Could you check a few things on this model? Use its own coordinates, in mm. A direction names the side the tool comes from. Give positions to 0.01 mm unless a question says otherwise; leave off trailing zeros. Order: outer loops, then holes, each group sorted by start corner. A loop starts at its lowest first (then second) coordinate and runs counter-clockwise, first axis right, second up. Notation, with made-up numbers: (24, 64) - (62, 64) arc R35 ccw to (62, 96) - close; hole circle Ø5 at (89.5, -22.75). An arc over 180 degrees is marked (long way). Put each result on its own line as item: value.
from build123d import *

# Parameters (mm, degrees)
SKETCH1_W           = 100
SKETCH1_H           = 40
BOSS_EXTRUDE1_DEPTH = 38
CUT_EXTRUDE2_START  = -12
SKETCH2_W           = 39.5
SKETCH2_H           = 34
CUT_EXTRUDE2_DEPTH  = 21
CUT_EXTRUDE4_REACH  = 81.36
SKETCH4_R           = 1.45
SKETCH6_W           = 100
SKETCH6_H           = 19
CUT_EXTRUDE5_DEPTH  = 87.215210375
FILLET1_R           = 0.5
CUT_EXTRUDE6_START  = 6.5
CUT_EXTRUDE6_DEPTH  = 0.5
CUT_EXTRUDE6_TAPER  = 2
CUT_EXTRUDE7_START  = 6.5
CUT_EXTRUDE7_DEPTH  = 0.5
CUT_EXTRUDE7_TAPER  = 2
CUT_EXTRUDE12_DEPTH = 9
CUT_EXTRUDE13_REACH = 72.385
SKETCH18_R          = 2.506862912
SKETCH18_R_2        = 2.693115416
SKETCH19_R          = 6.477
SKETCH19_R_2        = 4.572
CUT_EXTRUDE14_DEPTH = 0.79375


with BuildPart() as part:
    # Sketch1 → Boss-Extrude1 (new body)
    with BuildSketch(Plane.XY):
        with Locations((16.25, 1.5625)):
            Rectangle(SKETCH1_W, SKETCH1_H)
    extrude(amount=BOSS_EXTRUDE1_DEPTH)

    # Sketch2 → Cut-Extrude2 (cut)
    with BuildSketch(Plane(origin=(0, 0, 0), x_dir=(-1, 0, 0), z_dir=(0, 0, -1)).offset(CUT_EXTRUDE2_START)):
        with Locations((-38.5, 1.5625)):
            Rectangle(SKETCH2_W, SKETCH2_H)
        with Locations((6, 1.5625)):
            Rectangle(SKETCH2_W, SKETCH2_H)
    extrude(amount=-CUT_EXTRUDE2_DEPTH, mode=Mode.SUBTRACT)

    # Sketch4 → Cut-Extrude4 (cut, up to next)
    with BuildSketch(Plane(origin=(0, 0, 0), x_dir=(-1, 0, 0), z_dir=(0, 0, -1)), mode=Mode.PRIVATE) as cut_extrude4_sk1:
        with Locations((-62.25, 11.98479819)):
            Circle(SKETCH4_R)
    cut_extrude4_tool1 = extrude(cut_extrude4_sk1.sketch, amount=-CUT_EXTRUDE4_REACH, mode=Mode.PRIVATE) & part.part
    # Sketch4 → Cut-Extrude4 (cut, up to next)
    with BuildSketch(Plane(origin=(0, 0, 0), x_dir=(-1, 0, 0), z_dir=(0, 0, -1)), mode=Mode.PRIVATE) as cut_extrude4_sk2:
        with Locations((-62.25, -9.616561755)):
            Circle(SKETCH4_R)
    cut_extrude4_tool2 = extrude(cut_extrude4_sk2.sketch, amount=-CUT_EXTRUDE4_REACH, mode=Mode.PRIVATE) & part.part
    # Sketch4 → Cut-Extrude4 (cut, up to next)
    with BuildSketch(Plane(origin=(0, 0, 0), x_dir=(-1, 0, 0), z_dir=(0, 0, -1)), mode=Mode.PRIVATE) as cut_extrude4_sk3:
        with Locations((29.75, 11.98479819)):
            Circle(SKETCH4_R)
    cut_extrude4_tool3 = extrude(cut_extrude4_sk3.sketch, amount=-CUT_EXTRUDE4_REACH, mode=Mode.PRIVATE) & part.part
    # Sketch4 → Cut-Extrude4 (cut, up to next)
    with BuildSketch(Plane(origin=(0, 0, 0), x_dir=(-1, 0, 0), z_dir=(0, 0, -1)), mode=Mode.PRIVATE) as cut_extrude4_sk4:
        with Locations((29.75, -9.616561755)):
            Circle(SKETCH4_R)
    cut_extrude4_tool4 = extrude(cut_extrude4_sk4.sketch, amount=-CUT_EXTRUDE4_REACH, mode=Mode.PRIVATE) & part.part
    add(cut_extrude4_tool1.solids().sort_by_distance((62.25, 11.984798, 0))[0], mode=Mode.SUBTRACT)
    add(cut_extrude4_tool2.solids().sort_by_distance((62.25, -9.616562, 0))[0], mode=Mode.SUBTRACT)
    add(cut_extrude4_tool3.solids().sort_by_distance((-29.75, 11.984798, 0))[0], mode=Mode.SUBTRACT)
    add(cut_extrude4_tool4.solids().sort_by_distance((-29.75, -9.616562, 0))[0], mode=Mode.SUBTRACT)

    # Sketch6 → Cut-Extrude5 (cut, through all)
    with BuildSketch(Plane(origin=(0, 21.5625, 0), x_dir=(1, 0, 0), z_dir=(0, 1, 0))):
        with Locations((16.25, -28.5)):
            Rectangle(SKETCH6_W, SKETCH6_H)
    extrude(amount=-CUT_EXTRUDE5_DEPTH, mode=Mode.SUBTRACT)

    # Fillet1
    fillet1_edges = [part.edges().sort_by_distance(p)[0] for p in [
        (-25.75, -15.4375, 15.5),
        (13.75, -15.4375, 15.5),
        (-25.75, 18.5625, 15.5),
        (13.75, 18.5625, 15.5),
        (18.75, -15.4375, 15.5),
        (58.25, -15.4375, 15.5),
        (18.75, 18.5625, 15.5),
        (58.25, 18.5625, 15.5),
    ]]
    fillet(fillet1_edges, radius=FILLET1_R)

    # Sketch10 → Cut-Extrude6 (cut)
    with BuildSketch(Plane.XY.offset(12).offset(CUT_EXTRUDE6_START)):
        with BuildLine():
            Line((14.25, -14.9375), (14.25, 18.0625))
            ThreePointArc((14.25, 18.0625), (13.957106781, 18.769606781), (13.25, 19.0625))
            Line((13.25, 19.0625), (-25.25, 19.0625))
            ThreePointArc((-25.25, 19.0625), (-25.957106781, 18.769606781), (-26.25, 18.0625))
            Line((-26.25, 18.0625), (-26.25, -14.9375))
            ThreePointArc((-26.25, -14.9375), (-25.957106781, -15.644606781), (-25.25, -15.9375))
            Line((-25.25, -15.9375), (13.25, -15.9375))
            ThreePointArc((13.25, -15.9375), (13.957106781, -15.644606781), (14.25, -14.9375))
        make_face()
    extrude(amount=CUT_EXTRUDE6_DEPTH, taper=CUT_EXTRUDE6_TAPER, mode=Mode.SUBTRACT)

    # Sketch11 → Cut-Extrude7 (cut)
    with BuildSketch(Plane.XY.offset(12).offset(CUT_EXTRUDE7_START)):
        with BuildLine():
            Line((58.75, -14.9375), (58.75, 18.0625))
            ThreePointArc((58.75, 18.0625), (58.457106781, 18.769606781), (57.75, 19.0625))
            Line((57.75, 19.0625), (19.25, 19.0625))
            ThreePointArc((19.25, 19.0625), (18.542893219, 18.769606781), (18.25, 18.0625))
            Line((18.25, 18.0625), (18.25, -14.9375))
            ThreePointArc((18.25, -14.9375), (18.542893219, -15.644606781), (19.25, -15.9375))
            Line((19.25, -15.9375), (57.75, -15.9375))
            ThreePointArc((57.75, -15.9375), (58.457106781, -15.644606781), (58.75, -14.9375))
        make_face()
    extrude(amount=CUT_EXTRUDE7_DEPTH, taper=CUT_EXTRUDE7_TAPER, mode=Mode.SUBTRACT)

    # Sketch17 → Cut-Extrude12 (cut)
    with BuildSketch(Plane(origin=(0, 0, 0), x_dir=(-1, 0, 0), z_dir=(0, 0, -1))):
        with BuildLine():
            Line((-56.25, 9.0625), (23.75, 9.0625))
            ThreePointArc((23.75, 9.0625), (31.25, 1.5625), (23.75, -5.9375))
            Line((23.75, -5.9375), (-56.25, -5.9375))
            ThreePointArc((-56.25, -5.9375), (-63.75, 1.5625), (-56.25, 9.0625))
        make_face()
    extrude(amount=-CUT_EXTRUDE12_DEPTH, mode=Mode.SUBTRACT)

    # Sketch18 → Cut-Extrude13 (cut, up to next)
    with BuildSketch(Plane(origin=(0, 0, 9), x_dir=(-1, 0, 0), z_dir=(0, 0, -1)), mode=Mode.PRIVATE) as cut_extrude13_sk1:
        with Locations((-26.25, 1.5625)):
            Circle(SKETCH18_R)
    cut_extrude13_tool1 = extrude(cut_extrude13_sk1.sketch, amount=-CUT_EXTRUDE13_REACH, mode=Mode.PRIVATE) & part.part
    # Sketch18 → Cut-Extrude13 (cut, up to next)
    with BuildSketch(Plane(origin=(0, 0, 9), x_dir=(-1, 0, 0), z_dir=(0, 0, -1)), mode=Mode.PRIVATE) as cut_extrude13_sk2:
        with Locations((-6.25, 1.5625)):
            Circle(SKETCH18_R_2)
    cut_extrude13_tool2 = extrude(cut_extrude13_sk2.sketch, amount=-CUT_EXTRUDE13_REACH, mode=Mode.PRIVATE) & part.part
    add(cut_extrude13_tool1.solids().sort_by_distance((26.25, 1.5625, 9))[0], mode=Mode.SUBTRACT)
    add(cut_extrude13_tool2.solids().sort_by_distance((6.25, 1.5625, 9))[0], mode=Mode.SUBTRACT)

    # Sketch19 → Cut-Extrude14 (cut)
    # profile 1 of 2: a face of its own
    with BuildSketch(Plane(origin=(0, 0, 9), x_dir=(-1, 0, 0), z_dir=(0, 0, -1))):
        with Locations((-26.25, 1.5625)):
            Circle(SKETCH19_R)
        with Locations((-26.25, 1.5625)):
            Circle(SKETCH19_R_2, mode=Mode.SUBTRACT)
    # profile 2 of 2: a face of its own
    with BuildSketch(Plane(origin=(0, 0, 9), x_dir=(-1, 0, 0), z_dir=(0, 0, -1))):
        with Locations((-6.25, 1.5625)):
            Circle(SKETCH19_R)
        with Locations((-6.25, 1.5625)):
            Circle(SKETCH19_R_2, mode=Mode.SUBTRACT)
    extrude(amount=-CUT_EXTRUDE14_DEPTH, mode=Mode.SUBTRACT)


solid = part.part
1) Suppose I cut it at C-C, the plane z = 6. List the corners of the cut face in (x, y) for me.
Filled in:
outline: (-33.75, -18.44) - (66.25, -18.44) - (66.25, 21.56) - (-33.75, 21.56) - close; hole circle Ø2.9 at (-29.75, -9.62); hole circle Ø2.9 at (-29.75, 11.98); hole (-23.75, -5.94) - (56.25, -5.94) arc R7.5 ccw to (56.25, 9.06) - (-23.75, 9.06) arc R7.5 ccw to start; hole circle Ø2.9 at (62.25, -9.62); hole circle Ø2.9 at (62.25, 11.98)
2) Suppose I cut it at B-B, the plane x = 62.25. List the corners of the cut face in (y, z) for me, and give its area (3 significant figures).
Filled in:
outline: (-18.44, 0) - (-11.07, 0) - (-11.07, 19) - (-18.44, 19) - close; (-8.17, 0) - (-2.94, 0) - (-2.94, 9) - (6.06, 9) - (6.06, 0) - (10.53, 0) - (10.53, 19) - (-8.17, 19) - close; (13.43, 0) - (21.56, 0) - (21.56, 19) - (13.43, 19) - close
area: 569 mm^2
3) I'm going to push flat-ended pins straight in: pin 1 (1 mm diameter, centred on x = 55, y = 13.5, fed in from -Z); pin 2 (2.5 mm diameter, centred on x = -29.75, y = -9.62, fed in from -Z); pin 3 (6.5 mm diameter, centred on x = 26, y = -1.5, fed in from -Z); pin 4 (10 mm diameter, centred on x = 40.5, y = -3, fed in from +Z). Where does each tip first touch, or does it pass through?
Filled in:
pin 1: stops at z = 0
pin 2: passes through
pin 3: stops at z = 9
pin 4: stops at z = 12
4) If I drill on line 1 (X direction, y = -14, z = 17.75); line 2 (Y direction, x = 47, z = 17.75); line 3 (Y direction, x = 62.25, z = 8.75), over which ranges is the centre line in solid material (lowest first)? Write a range as [from, to].
Filled in:
line 1: x = [-33.75, -25.75], [13.75, 18.75], [58.25, 66.25]
line 2: y = [-18.44, -15.44], [18.56, 21.56]
line 3: y = [-18.44, -11.07], [-8.17, -2.94], [6.06, 10.53], [13.43, 21.56]
5) Which directions (+Z, -Z, +X, -X, +Y, -Y) give clear straight access to the entire face, cutting with the end or side of a thin tool? Please do faces 1 (the cylindrical face through (22.027, -0.189, 9.391)), 2 (the flat face through (-25.75, 1, 15)), 3 (the cylindrical face through (-31.133, -9.181, 9.367)).
Filled in:
face 1: -Z
face 2: +Z
face 3: +Z, -Z
6) Suppose I cut it at D-D, the plane x = 26.25. List the corners of the cut face in (y, z) for me, and give its area (3 significant figures).
Filled in:
outline: (-18.44, 0) - (-5.94, 0) - (-5.94, 9) - (-4.91, 9) - (-4.91, 9.79) - (-3.01, 9.79) - (-3.01, 9) - (-0.94, 9) - (-0.94, 12) - (-15.44, 12) - (-15.44, 18.5) - (-15.94, 18.5) - (-15.92, 19) - (-18.44, 19) - close; (4.07, 9) - (6.13, 9) - (6.13, 9.79) - (8.04, 9.79) - (8.04, 9) - (9.06, 9) - (9.06, 0) - (21.56, 0) - (21.56, 19) - (19.05, 19) - (19.06, 18.5) - (18.56, 18.5) - (18.56, 12) - (4.07, 12) - close
area: 368 mm^2
7) Suppose I cut it at A-A, the plane x = 6.25. List the corners of the cut face in (y, z) for me.
Filled in:
outline: (-18.44, 0) - (-5.94, 0) - (-5.94, 9) - (-4.91, 9) - (-4.91, 9.79) - (-3.01, 9.79) - (-3.01, 9) - (-1.13, 9) - (-1.13, 12) - (-15.44, 12) - (-15.44, 18.5) - (-15.94, 18.5) - (-15.92, 19) - (-18.44, 19) - close; (4.26, 9) - (6.13, 9) - (6.13, 9.79) - (8.04, 9.79) - (8.04, 9) - (9.06, 9) - (9.06, 0) - (21.56, 0) - (21.56, 19) - (19.05, 19) - (19.06, 18.5) - (18.56, 18.5) - (18.56, 12) - (4.26, 12) - close
8) We'd pull the mould along X, two halves only. Please class faces 4 (the flat face through (-33.75, 1, 9)), 5 (the cylindrical face through (63.7, 12, 9.4)), 6 (the flat face through (13.75, 1, 15)), 7 (the flat face through (16, 2, 19)): pulls with the +X half, pulls with the -X half, needs draft (parallel to the pull), parting line crosses it, or undercut.
Filled in:
face 4: pulls with the -X half
face 5: undercut
face 6: undercut
face 7: needs draft
